Can you work these out from the model? Positions are in its coordinate system, mm. Face numbers are marked on the shaded views. A direction names the side the tool comes from. Coordinates: 2 decimals unless noted, no trailing zeros. Loops run counter-clockwise (first coordinate to the right, second up) from the corner with the lowest first, then second, coordinate; pieces in that order, holes last. Notation, with made-up numbers: (-6, 77.25) -> (41, 77.25) arc R17 cw to (41, 104.25) -> close; hole circle Ø1 at (-23.75, 68). An arc over 180 degrees is marked (long way). Use one line per item in the form item = value. Start each with the question number.
(1) Imagine slicing it at D-D (z = 11). State how many separate pieces and enclosed holes the cut face has, plus the area to 3 significant figures.
(2) Thinking about a two-plate mould opening in Y: for the marked faces 6, 7, 8 and 9, which applies, released by +Y, released by -Y, zero draft, split by the parting line, or undercut?
(3) Imagine slicing it at B-B (y = -8). List the corners of the cut face in (x, z) for me, plus the area to 3 significant figures.
(4) Imagine slicing it at C-C (x = 8.5). List the corners of the cut face in (y, z) for me.
(5) On a 3-axis mill with a long thin cutter (end or side, diameter ignored), from which of +Z, -Z, +X, -X, +Y, -Y can I reach the whole of each face in a straight line? I mean the marked faces 1, 2, 3, 4 and 5. Say none if no direction works.
(6) I need wall thicknesses on line 1 (Y direction, x = 0, z = 13); line 2 (X direction, y = 1, z = 17.75); line 3 (X direction, y = -15.5, z = 13.25). Which ranges of each line are inside material? Lowest first, please. Write a range as [from, to].
(7) I'm going to push flat-ended pins straight in: pin 1 (12 mm diameter, centred on x = -2, y = -4.5, fed in from -Z); pin 2 (3 mm diameter, centred on y = -20, z = 11, fed in from +X); pin 3 (4 mm diameter, centred on y = -11.5, z = 20, fed in from +X); pin 4 (1.5 mm diameter, centred on x = 11, z = 10, fed in from +Y). Where does each tip first touch, or does it pass through?
(8) Imagine slicing it at A-A (x = 0). List the corners of the cut face in (y, z) for me.
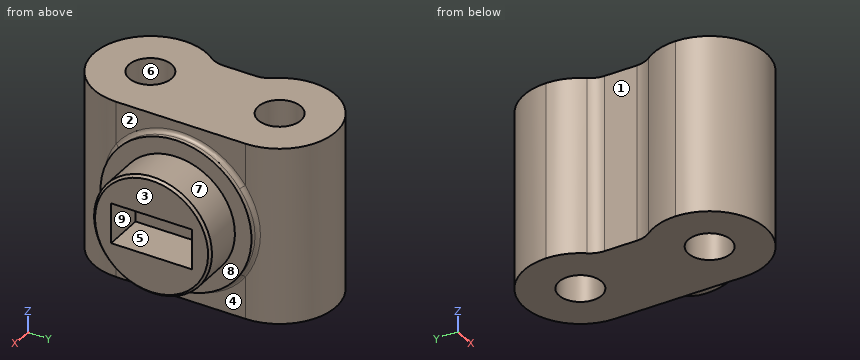
```python
from build123d import *

# Parameters (mm, degrees)
SKETCH_1_R           = 2.65
EXTRUDE_1_DEPTH      = 22
CUT_EXTRUDE_1_DEPTH  = 23
SKETCH_3_R           = 9.35
EXTRUDE_2_DEPTH      = 1
EXTRUDE_2_DEPTH_BACK = 1
SKETCH_4_R           = 7.3
EXTRUDE_3_DEPTH      = 5
CHAMFER_1_SIZE       = 0.3
SKETCH_5_W           = 5
SKETCH_5_H           = 10
CUT_EXTRUDE_2_DEPTH  = 5
FILLET_1_R           = 0.5


with BuildPart() as part:
    # 草图1 → 凸台-拉伸1 (new body)
    with BuildSketch(Plane.XY):
        with BuildLine():
            Line((-7, 0), (-7, -16))
            ThreePointArc((-7, -16), (0, -23), (7, -16))
            Line((7, -16), (7, 0))
            ThreePointArc((7, 0), (0, 7), (-7, 0))
        make_face()
        Circle(SKETCH_1_R, mode=Mode.SUBTRACT)
        with Locations((0, -16)):
            Circle(SKETCH_1_R, mode=Mode.SUBTRACT)
    extrude(amount=EXTRUDE_1_DEPTH)

    # 草图2 → 切除-拉伸1 (cut, through all)
    with BuildSketch(Plane.XY.offset(22)):
        with BuildLine():
            Line((-5, -6), (-5, -10))
            ThreePointArc((-5, -10), (-5.153950106, -10.948683298), (-5.6, -11.8))
            ThreePointArc((-5.6, -11.8), (-6.640783086, -13.786405638), (-7, -16))
            Line((-7, -16), (-7, 0))
            ThreePointArc((-7, 0), (-6.640783086, -2.213594362), (-5.6, -4.2))
            ThreePointArc((-5.6, -4.2), (-5.153950106, -5.051316702), (-5, -6))
        make_face()
    extrude(amount=-CUT_EXTRUDE_1_DEPTH, mode=Mode.SUBTRACT)

    # 草图3 → 凸台-拉伸2 (add, two sides)
    with BuildSketch(Plane(origin=(7, 0, 0), x_dir=(0, 0, -1), z_dir=(1, 0, 0))) as extrude_2_sk:
        with Locations((-11, -8)):
            Circle(SKETCH_3_R)
    extrude(amount=EXTRUDE_2_DEPTH)
    extrude(extrude_2_sk.sketch, amount=-EXTRUDE_2_DEPTH_BACK)

    # 草图4 → 凸台-拉伸3 (add)
    with BuildSketch(Plane(origin=(8, 0, 0), x_dir=(0, 0, -1), z_dir=(1, 0, 0))):
        with Locations((-11, -8)):
            Circle(SKETCH_4_R)
    extrude(amount=EXTRUDE_3_DEPTH)

    # 倒角1
    chamfer_1_edges = [part.edges().sort_by_distance(p)[0] for p in [
        (13, -8, 18.3),
    ]]
    chamfer(chamfer_1_edges, length=CHAMFER_1_SIZE)

    # 草图5 → 切除-拉伸2 (cut)
    with BuildSketch(Plane(origin=(13, 0, 0), x_dir=(0, 0, -1), z_dir=(1, 0, 0))):
        with Locations((-11, -8)):
            Rectangle(SKETCH_5_W, SKETCH_5_H)
    extrude(amount=-CUT_EXTRUDE_2_DEPTH, mode=Mode.SUBTRACT)

    # 圆角1
    fillet_1_edges = [part.edges().sort_by_distance(p)[0] for p in [
        (7, -8, 20.35),
        (-7, -16, 11),
        (7, -3.408078049, 2.855262264),
        (6.868587919, 1.35, 11),
    ]]
    fillet(fillet_1_edges, radius=FILLET_1_R)


solid = part.part
```
Worked out:
q1.separate_pieces = 1
q1.enclosed_holes = 2
q1.area = 357 mm2
q2.face_6 = undercut
q2.face_7 = split by the parting line
q2.face_8 = zero draft
q2.face_9 = undercut
q3.outline = (-5, 0) -> (7, 0) -> (7, 1.15) arc R0.5 cw to (7.5, 1.65) -> (8, 1.65) -> (8, 3.7) -> (12.7, 3.7) -> (13, 4) -> (13, 8.5) -> (8, 8.5) -> (8, 13.5) -> (13, 13.5) -> (13, 18) -> (12.7, 18.3) -> (8, 18.3) -> (8, 20.35) -> (7.5, 20.35) arc R0.5 cw to (7, 20.85) -> (7, 22) -> (-5, 22) -> close
q3.area = 331 mm2
q4.outline = circle Ø14.6 at (-8, 11); hole (-13, 8.5) -> (-3, 8.5) -> (-3, 13.5) -> (-13, 13.5) -> close
q5.face_1 = +Z, -Z, -X
q5.face_2 = +Z, +X
q5.face_3 = +Z, -Z, +X, +Y, -Y
q5.face_4 = -Z, +X
q5.face_5 = +X
q6.line_1 = [-23, -18.65], [-13.35, -2.65], [2.65, 7]
q6.line_2 = [-6.93, -2.45], [2.45, 6.93]
q6.line_3 = [-6.98, -2.6], [2.6, 8]
q7.pin_1 = 0
q7.pin_2 = 6.54
q7.pin_3 = 8
q7.pin_4 = -0.7
q8.outline = (-23, 0) -> (-18.65, 0) -> (-18.65, 22) -> (-23, 22) -> close; (-13.35, 0) -> (-2.65, 0) -> (-2.65, 22) -> (-13.35, 22) -> close; (2.65, 0) -> (7, 0) -> (7, 22) -> (2.65, 22) -> close
